Geometry: final body of the model. Coordinates: model frame, mm. Give positions to 0.01 mm unless a question says otherwise; leave off trailing zeros. Write each loop counter-clockwise with the first axis right and the second up, starting at its lowest first coordinate (ties: lowest second). Pieces come first, ordered by that corner, then holes.
from build123d import *

# Parameters (mm, degrees)
SKETCH1_W           = 406.4
SKETCH1_H           = 76.2
BOSS_EXTRUDE1_DEPTH = 50.8
SKETCH3_R           = 9.525
CUT_EXTRUDE1_DEPTH  = 50.8
SKETCH4_R           = 6.35
CUT_EXTRUDE2_DEPTH  = 8.89


with BuildPart() as part:
    # Sketch1 → Boss-Extrude1 (new body)
    with BuildSketch(Plane(origin=(0, 0, 0), x_dir=(1, 0, 0), z_dir=(0, 1, 0))):
        Rectangle(SKETCH1_W, SKETCH1_H)
    extrude(amount=BOSS_EXTRUDE1_DEPTH)

    # Sketch3 → Cut-Extrude1 (cut)
    with BuildSketch(Plane(origin=(0, 50.8, 0), x_dir=(1, 0, 0), z_dir=(0, 1, 0))):
        with Locations(Location((87.3125, 0, 0), (0, 0, 270))):
            Circle(SKETCH3_R)
    cut_extrude1 = extrude(amount=-CUT_EXTRUDE1_DEPTH, mode=Mode.SUBTRACT)

    # Sketch4 → Cut-Extrude2 (cut)
    with BuildSketch(Plane(origin=(0, 50.8, 0), x_dir=(1, 0, 0), z_dir=(0, 1, 0))):
        with Locations(Location((38.1, 25.4, 0), (0, 0, 270))):
            Circle(SKETCH4_R)
    cut_extrude2 = extrude(amount=-CUT_EXTRUDE2_DEPTH, mode=Mode.SUBTRACT)

    # Mirror1: Cut-Extrude1, Cut-Extrude2 across plane
    add(cut_extrude1.mirror(Plane(origin=(0, 0, 0), x_dir=(0, 0, 1), z_dir=(1, 0, 0))), mode=Mode.SUBTRACT)
    add(cut_extrude2.mirror(Plane(origin=(0, 0, 0), x_dir=(0, 0, 1), z_dir=(1, 0, 0))), mode=Mode.SUBTRACT)


solid = part.part
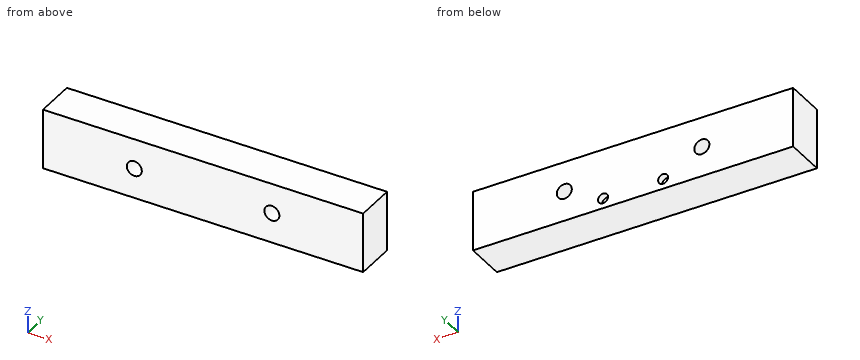
Q1. Ray query, line 1 along X through (y, z) = (24, 0); line 2 along X through (y, z) = (48.75, -25.4); line 3 along Z through (x, y) = (-38.1, 44.25). Return the intervals inside material, ascending.
Filled sheet:
line 1: x = -203.2 to -96.84, -77.79 to 77.79, 96.84 to 203.2
line 2: x = -203.2 to -44.45, -31.75 to 31.75, 44.45 to 203.2
line 3: z = -38.1 to -31.75, -19.05 to 38.1
Q2. Section A-A on z = 0. Output: boundary loops of the cut face in (x, y), plus the area to 3 significant figures.
Filled sheet:
outline: (-203.2, 0) - (-96.84, 0) - (-96.84, 50.8) - (-203.2, 50.8) - close; (-77.79, 0) - (77.79, 0) - (77.79, 50.8) - (-77.79, 50.8) - close; (96.84, 0) - (203.2, 0) - (203.2, 50.8) - (96.84, 50.8) - close
area: 18,700 mm2
Q3. Pin query (flat end, axial travel): P1, Ø6.5, axis at x = 39, z = -27, coming from the +Y side. Return the tip coordinate at first contact, or that it passes through.
Filled sheet:
P1: stops at y = 41.91
Q4. Section B-B on x = -38.1. Output: boundary loops of the cut face in (y, z).
Filled sheet:
outline: (0, -38.1) - (50.8, -38.1) - (50.8, -31.75) - (41.91, -31.75) - (41.91, -19.05) - (50.8, -19.05) - (50.8, 38.1) - (0, 38.1) - close
Q5. Section C-C on y = 30. Count the separate pieces of the cut face and the enclosed holes in it, plus the area to 3 significant figures.
Filled sheet:
separate pieces: 1
enclosed holes: 2
area: 30,400 mm2
